from build123d import *

# Parameters (mm, degrees)
F0_W      = 254
F0_H      = 254
F0_W_2    = 19.9865185836
F0_H_2    = 80.453767086
F1_DEPTH  = 1
F2_W      = 10
F2_H      = 8.3321671046
F3_DEPTH  = 16
F4_W      = 10
F4_H      = 8.3321671046
F4_R      = 4
F5_DEPTH  = 5
F6_W      = 7.4782028049
F6_H      = 8.1982985139
F7_DEPTH  = 11
F8_DEPTH  = 5
F11_R     = 4
F12_R     = 4
F9_R      = 2.5
F13_DEPTH = 5


with BuildPart() as f1:
    # F0 (on Front) → F1 (new body)
    with BuildSketch(Plane.XZ):
        with Locations((193.7753074374, -446.9196461141)):
            Rectangle(F0_W, F0_H)
        with Locations((130.3308923814, -466.3652455825)):
            Rectangle(F0_W_2, F0_H_2, mode=Mode.SUBTRACT)
    extrude(amount=F1_DEPTH)


with BuildPart() as f3:
    # F2 (on Top) → F3 (new body)
    with BuildSketch(Plane.XY):
        Rectangle(F2_W, F2_H)
    extrude(amount=F3_DEPTH)

    # F4 (on face) → F5 (cut)
    with BuildSketch(Plane.XY.offset(16)):
        Rectangle(F4_W, F4_H)
        Circle(F4_R, mode=Mode.SUBTRACT)
    extrude(amount=-F5_DEPTH, mode=Mode.SUBTRACT)

    # F6 (on face) → F7 (cut)
    with BuildSketch(Plane.XZ.offset(4.1660835523)):
        with Locations((1.2608985975, 4.0991492569)):
            Rectangle(F6_W, F6_H)
    extrude(amount=-F7_DEPTH, mode=Mode.SUBTRACT)

    # F8 (add): a face of the model
    f8_faces = [f3.faces().sort_by_distance(p)[0] for p in [
        (0, 0, 16),
    ]]
    extrude(f8_faces, amount=F8_DEPTH)

    # F11
    f11_edges = [f3.edges().sort_by_distance(p)[0] for p in [
        (-4, 0, 21),
    ]]
    fillet(f11_edges, radius=F11_R)

    # F12
    f12_edges = [f3.edges().sort_by_distance(p)[0] for p in [
        (-3.739101, -4.166084, 0),
        (-3.739101, 4.166084, 0),
    ]]
    fillet(f12_edges, radius=F12_R)

    # F9 (on face) → F13 (cut)
    with BuildSketch(Plane.YZ.offset(-2.4782028049)):
        with Locations((0, 4.5)):
            Circle(F9_R)
    extrude(amount=-F13_DEPTH, mode=Mode.SUBTRACT)


solid = f3.part
Design review of the part built by this model. Coordinates are the model's own, in mm. A direction names the side the tool comes from. Coordinates: 2 decimals unless noted, no trailing zeros. Loops run counter-clockwise (first coordinate to the right, second up) from the corner with the lowest first, then second, coordinate; pieces in that order, holes last. Notation, with made-up numbers: M -9,-7 L 18,-7 A12 ccw 18,9 Z; hole C 79.25,22 d2. An arc over 180 degrees is marked long. Use one line per item in the form item = value.
(1) For line 1 along Z through (x, y) = (-4.4, 0); line 2 along X through (y, z) = (3.25, 5.75); line 3 along Z through (x, y) = (-2.25, 3.5), list the stretches that pass through material, from the lowest coordinate up. Write a range as from..to.
Return value:
line_1 = 0..2, 7..11
line_2 = -5..-2.48
line_3 = 8.2..11
(2) Consider section B-B (x = 0). Write out the cut boundary in (y, z), and give its area (3 significant figures).
Return value:
outline = M -4.17,8.2 L 4.17,8.2 L 4.17,11 L 4,11 L 4,17 A4 ccw -4,17 L -4,11 L -4.17,11 Z
area = 96.5 mm2
(3) Clearance check with flat-ended pins moving along their axes: P1, Ø1, axis at y = 0, z = 17.5, coming from the +X side; P2, Ø1.5, axis at y = -2, z = 5.5, coming from the -X side; P3, Ø2, axis at y = -3, z = 18, coming from the +X side; P4, Ø4, axis at x = 3, y = 1, coming from the -Z side. State where each tip first meets the part, or that it passes through.
Return value:
P1 = 4
P2 = -5
P3 = 3.37
P4 = 8.2
(4) For faces 4 (the face through (-2, -4, 11)), 5 (the face through (1, 0, 8.198)), 6 (the face through (-3.721, 3.025, 1.203)), list the 3-axis set-ups (+Z, -Z, +X, -X, +Y, -Y) from which the entire face can be reached by the end or side of a thin tool; tool diameter is ignored.
Return value:
face_4 = +Z
face_5 = -Z, +X, +Y, -Y
face_6 = -Z, +X, -X, +Y
(5) Consider section C-C (y = 1). Write out the cut boundary in (x, z).
Return value:
outline = M -5,0.09 L -2.48,0.09 L -2.48,2.21 L -5,2.21 Z; M -5,6.79 L -2.48,6.79 L -2.48,8.2 L 5,8.2 L 5,11 L 3.87,11 L 3.87,17 A3.87 ccw -3.87,17 L -3.87,11 L -5,11 Z
(6) Consider section A-A (z = 4.5). Write out the cut boundary in (x, y), and give its area (3 significant figures).
Return value:
outline = M -5,-4.17 L -2.48,-4.17 L -2.48,-2.5 L -5,-2.5 Z; M -5,2.5 L -2.48,2.5 L -2.48,4.17 L -5,4.17 Z
area = 8.40 mm2
(7) Draft analysis for pull direction Y (two halves, no side actions). For faces 1 (the face through (-4, 0, 7)), 2 (the face through (-1, 4.166, 9)), 3 (the face through (-0.867, -3.905, 14.042)), state which applies: pulls with the +Y half, pulls with the -Y half, needs draft (parallel to the pull), parting line crosses it, or undercut.
Return value:
face_1 = undercut
face_2 = pulls with the +Y half
face_3 = parting line crosses it
(8) Consider section D-D (x = -3.25). Write out the cut boundary in (y, z), and give its area (3 significant figures).
Return value:
outline = M -4.17,4 A4 ccw -0.17,0 L 0.17,0 A4 ccw 4.17,4 L 4.17,11 L 2.33,11 L 2.33,17 A2.33 ccw -2.33,17 L -2.33,11 L -4.17,11 Z; hole C 0,4.5 d5
area = 102 mm2
